Geometry check sheet. Reference: the model listing, model coordinates, mm. Face numbers are marked on the shaded views. Round coordinates to 2 decimals unless told otherwise and drop trailing zeros. Order: outer loops, then holes, each group sorted by start corner. A loop starts at its lowest first (then second) coordinate and runs counter-clockwise, first axis right, second up. Notation, with made-up numbers: (0.25, 3.5) - (37.25, 3.5) arc R26 ccw to (37.25, 33.5) - close; hole circle Ø4 at (33.25, 3). An arc over 180 degrees is marked (long way). Return JSON: item names as keys, results as strings. Group by question number.
Q1. Sectioned sample at B-B, the plane y = 0. Record the cut outline in (x, z), then the cut area to 3 significant figures.
Q2. Draft check along Y on the marked faces 1, 2, 3 and 4. Enter one of: pulls with the +Y half, pulls with the -Y half, needs draft (parallel to the pull), parting line crosses it, or undercut.
Q3. Gauge pin test, flat ends, axial feed: pin 1 Ø1.1 at (y, z) = (0, 2) entering from -X; pin 2 Ø8 at (x, y) = (-6, 7.5) entering from +Z; pin 3 Ø0.8 at (x, z) = (0.5, 2) entering from -Y. Record the tip position at first contact, or that the pin passes through.
Q4. Sectioned sample at D-D, the plane y = 5. Record the cut outline in (x, z).
Q5. Material ranges on line 1 along X through (y, z) = (0, 0.45); line 2 along Y through (x, z) = (0, 0.65); line 3 along Z through (x, y) = (2.5, 6.25), recorded low to high.
Q6. Sectioned sample at A-A, the plane x = 0. Record the cut outline in (y, z).
Q7. Sectioned sample at C-C, the plane z = 0.65. Record the cut outline in (x, y), then the cut area to 3 significant figures.
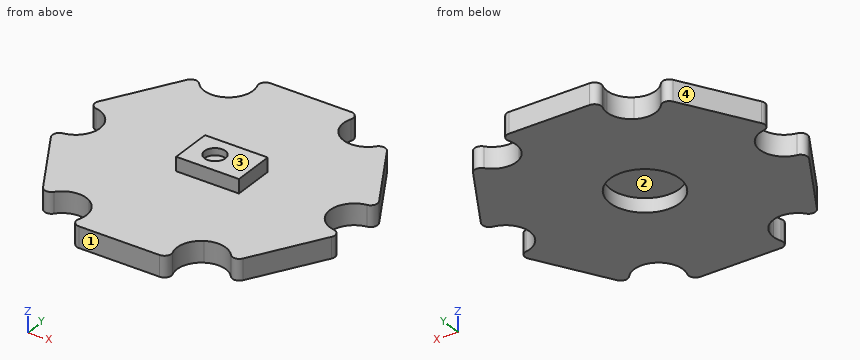
```python
from build123d import *

# Parameters (mm, degrees)
F1_DEPTH  = 1.5
F2_R      = 1.75
F3_DEPTH  = 25
F4_R      = 0.5
F5_R      = 2.5
F6_DEPTH  = 1
F7_W      = 4.5
F7_H      = 3
F8_DEPTH  = 1
F9_R      = 0.75
F10_DEPTH = 0.5


with BuildPart() as f1:
    # F0 (on Top) → F1 (new body)
    with BuildSketch(Plane.XY):
        Polygon((5.7504086811, 9.96), (-5.7504086811, 9.96), (-11.5008173623, 0), (-5.7504086811, -9.96), (5.7504086811, -9.96), (11.5008173623, 0), align=None)
    extrude(amount=F1_DEPTH)

    # F2 (on face) → F3 (cut)
    with BuildSketch(Plane.XY.offset(1.5)):
        with BuildLine():
            ThreePointArc((6.7504086811, 8.6609618943), (4.1254086811, 10.1765063509), (4.1254086811, 7.1454174377))
            ThreePointArc((4.1254086811, 7.1454174377), (5.8754086811, 7.1454174377), (6.7504086811, 8.6609618943))
        make_face()
        with BuildLine():
            ThreePointArc((11.7508173623, 0), (10.0008173623, 1.75), (8.2508173623, 0))
            ThreePointArc((8.2508173623, 0), (10.0008173623, -1.75), (11.7508173623, 0))
        make_face()
        with BuildLine():
            ThreePointArc((6.7504086811, -8.6609618943), (5.8754086811, -7.1454174377), (4.1254086811, -7.1454174377))
            ThreePointArc((4.1254086811, -7.1454174377), (4.1254086811, -10.1765063509), (6.7504086811, -8.6609618943))
        make_face()
        with BuildLine():
            ThreePointArc((-3.2504086811, -8.6609618943), (-3.4848642245, -7.7859618943), (-4.1254086811, -7.1454174377))
            ThreePointArc((-4.1254086811, -7.1454174377), (-6.5159531378, -9.5359618943), (-3.2504086811, -8.6609618943))
        make_face()
        with Locations((-10.0008173623, 0)):
            Circle(F2_R)
        with BuildLine():
            ThreePointArc((-3.2504086811, 8.6609618943), (-6.5159531378, 9.5359618943), (-4.1254086811, 7.1454174377))
            ThreePointArc((-4.1254086811, 7.1454174377), (-3.4848642245, 7.7859618943), (-3.2504086811, 8.6609618943))
        make_face()
    extrude(amount=-F3_DEPTH, mode=Mode.SUBTRACT)

    # F4
    f4_edges = [f1.edges().sort_by_distance(p)[0] for p in [
        (-3.827805, 9.96, 0.75),
        (-6.711711, 8.294976, 0.75),
        (3.827805, 9.96, 0.75),
        (6.711711, 8.294976, 0.75),
        (-10.539515, 1.665024, 0.75),
        (-10.539515, -1.665024, 0.75),
        (-3.827805, -9.96, 0.75),
        (-6.711711, -8.294976, 0.75),
        (3.827805, -9.96, 0.75),
        (6.711711, -8.294976, 0.75),
        (10.539515, 1.665024, 0.75),
        (10.539515, -1.665024, 0.75),
    ]]
    fillet(f4_edges, radius=F4_R)

    # F5 (on face) → F6 (cut)
    with BuildSketch(Plane(origin=(0, 0, 0), x_dir=(1, 0, 0), z_dir=(0, 0, -1))):
        Circle(F5_R)
    extrude(amount=-F6_DEPTH, mode=Mode.SUBTRACT)

    # F7 (on face) → F8 (join)
    with BuildSketch(Plane.XY.offset(1.5)):
        with Locations((0.5, 0)):
            Rectangle(F7_W, F7_H)
    extrude(amount=F8_DEPTH)

    # F9 (on face) → F10 (cut)
    with BuildSketch(Plane.XY.offset(2.5)):
        Circle(F9_R)
    extrude(amount=-F10_DEPTH, mode=Mode.SUBTRACT)


solid = f1.part
```
Reply:
{
 "1": {"outline": "(-8.25, 0) - (-2.5, 0) - (-2.5, 1) - (2.5, 1) - (2.5, 0) - (8.25, 0) - (8.25, 1.5) - (2.75, 1.5) - (2.75, 2.5) - (0.75, 2.5) - (0.75, 2) - (-0.75, 2) - (-0.75, 2.5) - (-1.75, 2.5) - (-1.75, 1.5) - (-8.25, 1.5) - close", "area": "23.5 mm^2"},
 "2": {"face 1": "pulls with the -Y half", "face 2": "undercut", "face 3": "needs draft", "face 4": "pulls with the +Y half"},
 "3": {"pin 1": "x = -8.27", "pin 2": "z = 1.5", "pin 3": "y = -1.5"},
 "4": {"outline": "(-8.61, 0) - (8.61, 0) - (8.61, 1.5) - (-8.61, 1.5) - close"},
 "5": {"line 1": "-8.25 to -2.5, 2.5 to 8.25", "line 2": "-9.96 to -2.5, 2.5 to 9.96", "line 3": "0 to 1.5"},
 "6": {"outline": "(-9.96, 0) - (-2.5, 0) - (-2.5, 1) - (2.5, 1) - (2.5, 0) - (9.96, 0) - (9.96, 1.5) - (1.5, 1.5) - (1.5, 2.5) - (0.75, 2.5) - (0.75, 2) - (-0.75, 2) - (-0.75, 2.5) - (-1.5, 2.5) - (-1.5, 1.5) - (-9.96, 1.5) - close"},
 "7": {"outline": "(-10.07, -2.47) - (-7.18, -7.49) arc R0.5 ccw to (-6.36, -7.55) arc R1.75 cw to (-3.36, -9.28) arc R0.5 ccw to (-2.9, -9.96) - (2.9, -9.96) arc R0.5 ccw to (3.36, -9.28) arc R1.75 cw to (6.36, -7.55) arc R0.5 ccw to (7.18, -7.49) - (10.07, -2.47) arc R0.5 ccw to (9.72, -1.73) arc R1.75 cw to (9.72, 1.73) arc R0.5 ccw to (10.07, 2.47) - (7.18, 7.49) arc R0.5 ccw to (6.36, 7.55) arc R1.75 cw to (3.36, 9.28) arc R0.5 ccw to (2.9, 9.96) - (-2.9, 9.96) arc R0.5 ccw to (-3.36, 9.28) arc R1.75 cw to (-6.36, 7.55) arc R0.5 ccw to (-7.18, 7.49) - (-10.07, 2.47) arc R0.5 ccw to (-9.72, 1.73) arc R1.75 cw to (-9.72, -1.73) arc R0.5 ccw to start; hole circle Ø5 at (0, 0)", "area": "272 mm^2"}
}
